Geometry check sheet. Reference: the model listing, model coordinates, mm. Round coordinates to 2 decimals unless told otherwise and drop trailing zeros. Loops run counter-clockwise (first coordinate to the right, second up) from the corner with the lowest first, then second, coordinate; pieces in that order, holes last. Notation, with made-up numbers: M 62,-20 L 67,-20 A13 ccw 67,-8 Z; hole C 76,2 d7. An arc over 180 degrees is marked long. Use one line per item in the form item = value. Start each with the question number.
1. Go/stop test with flat-tipped pins: pin 1 (2 mm diameter, centred on x = 9.5, y = 44, fed in from -Z); pin 2 (1 mm diameter, centred on x = 9.5, z = 122, fed in from +Y); pin 3 (1 mm diameter, centred on x = 4.5, y = 26.5, fed in from -Z). Record where each tip stops, or that it passes through.
2. Material ranges on line 1 (Z direction, x = 3, y = 11); line 2 (Y direction, x = 9.5, z = 104); line 3 (Y direction, x = 4.25, z = 82), recorded low to high.
3. Cross-section at C-C (z = 101). Record the boundary of the cut face in (x, y).
4. Cross-section at B-B (y = 103.5). Record the boundary of the cut face in (x, z).
5. Cross-section at A-A (x = 4.75). Record the boundary of the cut face in (y, z).
Autodesk Fusion 360 part; units mm, degrees
sketch "Name Sign Support" plane through (0, 0, 0) normal (1, 0, 0) x (0, 1, 0) in component "Name Sign Support (1)"
  line L0 (-0.0158, 97.2466) -> (88.3556, 61.0028)
  line L1 (163.2949, 85.69) -> (-0.0158, 152.6686)
  line L2 (-0.0158, 152.6686) -> (-0.0158, 97.2466)
  line L3 (163.2949, 85.69) -> (163.2949, 61.0028)
  line L4 (88.3556, 61.0028) -> (163.2949, 61.0028)
  dimension "d18" = 67.7
  dimension "d9" = 55.422
  dimension "d2" = 176.512
  dimension "d3" = 95.515
extrude "Extrude2" add sketch "Name Sign Support" along normal blind 12 in component "Name Sign Support (1)"
component "Name Sign Support Left" placed x (1, 0, 0) y (0, 1, 0) z (0, 0, 1) at (0, 0, 0)
component "Name Sign Support" placed x (1, 0, 0) y (0, 1, 0) z (0, 0, 1) at (0, 0, 0) in component "Name Sign Support Left"
component "Name Sign Support (1)" placed x (1, 0, 0) y (0, 1, 0) z (0, 0, 1) at (0, 0, 0) in component "Name Sign Support"
equation "d19 = pineThickness"
equation "pineThickness = 12 mm"
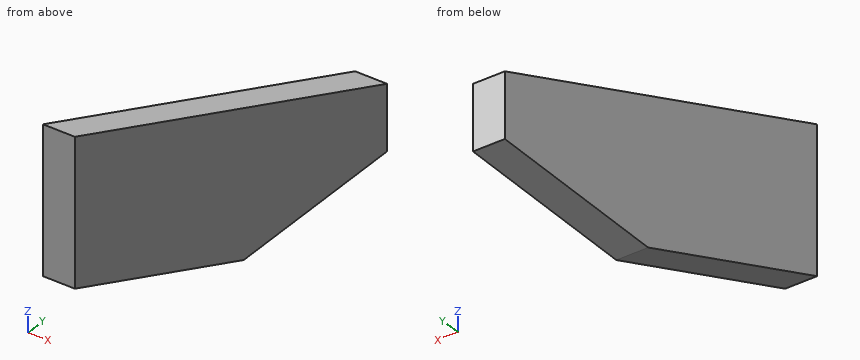
Reported:
q1.pin_1 = 78.78
q1.pin_2 = 75.98
q1.pin_3 = 86.17
q2.line_1 = 92.73 to 148.15
q2.line_2 = -0.02 to 118.65
q2.line_3 = 37.16 to 163.29
q3.outline = M 0,-0.02 L 12,-0.02 L 12,125.97 L 0,125.97 Z
q4.outline = M 0,61 L 12,61 L 12,110.21 L 0,110.21 Z
q5.outline = M -0.02,97.25 L 88.36,61 L 163.29,61 L 163.29,85.69 L -0.02,152.67 Z
